Geometry: final body of the model. Coordinates: model frame, mm. A direction names the side the tool comes from. Give positions to 0.01 mm unless a question says otherwise; leave off trailing zeros. Write each loop counter-clockwise with the first axis right and the second up, starting at its lowest first coordinate (ties: lowest second). Pieces come first, ordered by that corner, then holes.
Q1. Section B-B (x = 3). Return the cut outline in (y, z), plus the area to 3 significant figures.
Q2. Section C-C (y = 3.5). Return the cut outline in (x, z) (3 decimals), plus the area to 3 significant figures.
Q3. Line query: line 1 (X direction, y = -10.5, z = 7.25) (3 decimals); line 2 (X direction, y = -10.62, z = 3) (3 decimals); line 3 (X direction, y = -10.62, z = 11) (3 decimals). Output: solid intervals per line, ascending.
Q4. Section D-D (z = 4.75). Return the cut outline in (x, y) (3 decimals).
Q5. Pin query (flat end, axial travel): pin 1 Ø7 at (x, y) = (-15.5, -5) entering from +Z. Return the tip coordinate at first contact, or that it passes through.
Q6. Mould query, pull axis Y, two halves, no side actions, for faces 4 (the cylindrical face through (13.971, -11.906, 7.723)), 5 (the cylindrical face through (-14.581, 9.455, 5.269)), 6 (the cylindrical face through (-0.645, 0.196, 12.184)), 7 (the flat face through (4, 14, 11)). Classes: +Y half, -Y half, draft (parallel to the pull), parting line (faces both ways), or undercut.
Q7. Reachability of faces 1 (the flat face through (16.965, 0, 15)), 2 (the flat face through (-14, 0, 10.16)), 3 (the cylindrical face through (14.451, 9.984, 7.723)) from +Z, -Z, +X, -X, +Y, -Y: full face, straight path, thin tool, end or side. Return the list, or none.
Q8. Section A-A (z = 17.29). Return the cut outline in (x, y) (3 decimals), plus the area to 3 significant figures.
Autodesk Inventor part; units mm, degrees
ref_plane "YZ Plane" through (0, 0, 0) normal (1, 0, 0) x (0, 1, 0)
ref_plane "XZ Plane" through (0, 0, 0) normal (0, 1, 0) x (-1, 0, 0)
ref_plane "XY Plane" through (0, 0, 0) normal (0, 0, 1) x (1, 0, 0)
sketch "Sketch2" plane through (0, 0, 0) normal (0, 0, 1) x (1, 0, 0)
  line L0 (-16.965, 14) -> (16.965, 14)
  line L1 (16.965, 14) -> (16.965, -14)
  line L2 (16.965, -14) -> (-16.965, -14)
  line L3 (-16.965, -14) -> (-16.965, 14)
  line L4 (-16.965, 14) -> (16.965, -14) construction
  line L5 (16.965, 14) -> (-16.965, -14) construction
  point P0 (0, 0)
  dimension "d0" = 33.93
  dimension "d1" = 28
extrude "Extrusion1" add sketch "Sketch2" along normal blind 29.6
sketch "Sketch4" plane through (0, 0, 0) normal (0, 0, -1) x (-1, 0, 0)
  line L0 (16.965, 14) -> (16.965, -14) construction
  line L1 (-16.965, 14) -> (16.965, 14) construction
  line L2 (16.965, -14) -> (-16.965, -14) construction
  line L3 (-16.965, -14) -> (-16.965, 14) construction
  point P0 (13.485, 10.65)
  point P1 (13.665, -10.64)
  point P2 (-12.985, -10.62)
  point P3 (-13.465, 11.27)
  dimension "d11" = 3.48
  dimension "d12" = 3.3
  dimension "d13" = 3.35
  dimension "d14" = 3.36
  dimension "d15" = 3.38
  dimension "d16" = 3.98
  dimension "d17" = 3.5
  dimension "d18" = 2.73
hole "Hole1" at (13.465, 11.27, 0) at (12.985, -10.62, 0) at (-13.665, -10.64, 0) at (-13.485, 10.65, 0) direction (0, 0, 1) diameter 3.242 depth 15 tip angle 118
sketch "Sketch3" plane through (-16.965, 14, 0) normal (0, 1, 0) x (1, 0, 0)
  circle A0 centre (16.99, -17.29) radius 5.15
  line L0 (0, 0) -> (0, -29.6)
  line L1 (33.93, 0) -> (0, 0)
  line L2 (33.93, -29.6) -> (0, -29.6) construction
  line L3 (11.84, -12.14) -> (22.14, -12.14) construction
  line L4 (22.14, -12.14) -> (22.14, -22.44) construction
  line L5 (22.14, -22.44) -> (11.84, -22.44) construction
  line L6 (11.84, -22.44) -> (11.84, -12.14) construction
  line L7 (11.84, -12.14) -> (22.14, -22.44) construction
  line L8 (22.14, -12.14) -> (11.84, -22.44) construction
  line L9 (33.93, 0) -> (33.93, -29.6)
  point P0 (16.965, 0)
  point P1 (0, -14.8)
  point P2 (16.965, 0)
  dimension "d4" = 10.3
  dimension "d30" = 7.16
  dimension "d32" = 11.79
extrude "Extrusion2" cut sketch "Sketch3" against normal through all
sketch "Sketch5" plane through (-16.965, -14, 0) normal (-1, 0, 0) x (0, 0, 1)
  line L0 (29.6, 0) -> (29.6, 28)
  line L1 (22.44, 0) -> (12.14, 0)
  line L2 (29.6, 28) -> (10.16, 28)
  line L3 (10.16, 28) -> (10.16, 0)
  line L4 (10.16, 0) -> (29.6, 0)
  line L5 (29.6, 0) -> (29.6, 28)
  point P0 (0, 14)
  dimension "d26" = 19.44
extrude "Extrusion3" cut sketch "Sketch5" against normal blind 6.22
move faces "Move1" translate (0, 0, 0.24) faces at (3.877, 3.4597, 0)
properties part number "Upper Z lifter"
Computed:
1. outline: (-14, 0.24) - (14, 0.24) - (14, 13.09) - (-14, 13.09) - close; (-14, 21.49) - (14, 21.49) - (14, 29.6) - (-14, 29.6) - close
1. area: 587 mm2
2. outline: (-16.965, 0.24) - (16.965, 0.24) - (16.965, 29.6) - (-10.745, 29.6) - (-10.745, 10.16) - (-16.965, 10.16) - close; hole circle Ø10.3 at (0.025, 17.29)
2. area: 792 mm2
3. line 1: x = -16.965 to -15.28, -12.05 to 11.368, 14.602 to 16.965
3. line 2: x = -16.965 to -15.286, -12.044 to 11.364, 14.606 to 16.965
3. line 3: x = -10.745 to 11.364, 14.606 to 16.965
4. outline: (-16.965, -14) - (16.965, -14) - (16.965, 14) - (-16.965, 14) - close; hole circle Ø3.242 at (-13.665, -10.64); hole circle Ø3.242 at (-13.485, 10.65); hole circle Ø3.242 at (12.985, -10.62); hole circle Ø3.242 at (13.465, 11.27)
5. pin 1: stops at z = 10.16
6. face 4: undercut
6. face 5: undercut
6. face 6: draft
6. face 7: +Y half
7. face 1: +Z, -Z, +X, +Y, -Y
7. face 2: +Z, -X, +Y, -Y
7. face 3: -Z
8. outline: (-10.745, -14) - (-5.125, -14) - (-5.125, 14) - (-10.745, 14) - close; (5.175, -14) - (16.965, -14) - (16.965, 14) - (5.175, 14) - close
8. area: 487 mm2
